```python
from build123d import *

# Parameters (mm, degrees)
BOSS_EXTRUDE1_DEPTH                                = 9.5
BOSS_EXTRUDE2_DEPTH                                = 2
BOSS_EXTRUDE4_DEPTH                                = 11.5
BOSS_EXTRUDE6_DEPTH                                = 7.5
CUT_EXTRUDE1_DEPTH                                 = 2
CUT_EXTRUDE2_REACH                                 = 85.313
SKETCH9_W                                          = 10
SKETCH9_H                                          = 3
CHAMFER1_SIZE                                      = 1
CHAMFER2_SIZE                                      = 1
CBORE_FOR_M2_5_PAN_HEAD_MACHINE_SCREW1_D           = 2.9
CBORE_FOR_M2_5_PAN_HEAD_MACHINE_SCREW1_CBORE_D     = 6
CBORE_FOR_M2_5_PAN_HEAD_MACHINE_SCREW1_CBORE_DEPTH = 2.1
CBORE_FOR_M2_5_PAN_HEAD_MACHINE_SCREW2_D           = 2.9
CBORE_FOR_M2_5_PAN_HEAD_MACHINE_SCREW2_CBORE_D     = 6
CBORE_FOR_M2_5_PAN_HEAD_MACHINE_SCREW2_CBORE_DEPTH = 2.1
CBORE_FOR_M2_5_PAN_HEAD_MACHINE_SCREW3_D           = 2.9
CBORE_FOR_M2_5_PAN_HEAD_MACHINE_SCREW3_CBORE_D     = 6
CBORE_FOR_M2_5_PAN_HEAD_MACHINE_SCREW3_CBORE_DEPTH = 2.1
CBORE_FOR_M2_5_PAN_HEAD_MACHINE_SCREW4_D           = 2.9
CBORE_FOR_M2_5_PAN_HEAD_MACHINE_SCREW4_CBORE_D     = 6
CBORE_FOR_M2_5_PAN_HEAD_MACHINE_SCREW4_CBORE_DEPTH = 2.1
SKETCH18_W                                         = 54.5
SKETCH18_H                                         = 7.531088913
CUT_EXTRUDE3_DEPTH                                 = 2


with BuildPart() as part:
    # Sketch2 → Boss-Extrude1 (new body)
    with BuildSketch(Plane(origin=(0, 0, 0), x_dir=(1, 0, 0), z_dir=(0, 1, 0))):
        with BuildLine():
            Line((-30.346153846, 41.446848386), (27.653846154, 41.446848386))
            ThreePointArc((27.653846154, 41.446848386), (32.250040232, 39.543042463), (34.153846154, 34.946848386))
            Line((34.153846154, 34.946848386), (34.153846154, -34.053151614))
            ThreePointArc((34.153846154, -34.053151614), (32.250040232, -38.649345692), (27.653846154, -40.553151614))
            Line((27.653846154, -40.553151614), (-30.346153846, -40.553151614))
            ThreePointArc((-30.346153846, -40.553151614), (-34.942347924, -38.649345692), (-36.846153846, -34.053151614))
            Line((-36.846153846, -34.053151614), (-36.846153846, 34.946848386))
            ThreePointArc((-36.846153846, 34.946848386), (-34.942347924, 39.543042463), (-30.346153846, 41.446848386))
        make_face()
        with BuildLine():
            Line((-30.346153846, 39.446848386), (27.653846154, 39.446848386))
            ThreePointArc((27.653846154, 39.446848386), (30.835826669, 38.128828901), (32.153846154, 34.946848386))
            Line((32.153846154, 34.946848386), (32.153846154, -34.053151614))
            ThreePointArc((32.153846154, -34.053151614), (30.835826669, -37.23513213), (27.653846154, -38.553151614))
            Line((27.653846154, -38.553151614), (-30.346153846, -38.553151614))
            ThreePointArc((-30.346153846, -38.553151614), (-33.528134361, -37.23513213), (-34.846153846, -34.053151614))
            Line((-34.846153846, -34.053151614), (-34.846153846, 34.946848386))
            ThreePointArc((-34.846153846, 34.946848386), (-33.528134361, 38.128828901), (-30.346153846, 39.446848386))
        make_face(mode=Mode.SUBTRACT)
    extrude(amount=BOSS_EXTRUDE1_DEPTH)

    # Sketch3 → Boss-Extrude2 (add)
    with BuildSketch(Plane(origin=(0, 0, 0), x_dir=(1, 0, 0), z_dir=(0, 1, 0))):
        with BuildLine():
            Line((-30.346153846, -38.553151614), (27.653846154, -38.553151614))
            ThreePointArc((27.653846154, -38.553151614), (30.835826669, -37.23513213), (32.153846154, -34.053151614))
            Line((32.153846154, -34.053151614), (32.153846154, 34.946848386))
            ThreePointArc((32.153846154, 34.946848386), (30.835826669, 38.128828901), (27.653846154, 39.446848386))
            Line((27.653846154, 39.446848386), (-30.346153846, 39.446848386))
            ThreePointArc((-30.346153846, 39.446848386), (-33.528134361, 38.128828901), (-34.846153846, 34.946848386))
            Line((-34.846153846, 34.946848386), (-34.846153846, -34.053151614))
            ThreePointArc((-34.846153846, -34.053151614), (-33.528134361, -37.23513213), (-30.346153846, -38.553151614))
        make_face()
    extrude(amount=BOSS_EXTRUDE2_DEPTH)

    # Sketch6 → Boss-Extrude4 (add)
    with BuildSketch(Plane(origin=(0, 2, 0), x_dir=(1, 0, 0), z_dir=(0, 1, 0))):
        with BuildLine():
            Line((-26.846153846, 34.946848386), (-26.846153846, 39.446848386))
            Line((-26.846153846, 39.446848386), (-30.346153846, 39.446848386))
            ThreePointArc((-30.346153846, 39.446848386), (-33.528134361, 38.128828901), (-34.846153846, 34.946848386))
            Line((-34.846153846, 34.946848386), (-34.846153846, 31.446848386))
            Line((-34.846153846, 31.446848386), (-30.346153846, 31.446848386))
            ThreePointArc((-30.346153846, 31.446848386), (-27.871280112, 32.471974652), (-26.846153846, 34.946848386))
        make_face()
        with BuildLine():
            Line((24.153846154, 34.946848386), (24.153846154, 39.446848386))
            Line((24.153846154, 39.446848386), (27.653846154, 39.446848386))
            ThreePointArc((27.653846154, 39.446848386), (30.835826669, 38.128828901), (32.153846154, 34.946848386))
            Line((32.153846154, 34.946848386), (32.153846154, 31.446848386))
            Line((32.153846154, 31.446848386), (27.653846154, 31.446848386))
            ThreePointArc((27.653846154, 31.446848386), (25.17897242, 32.471974652), (24.153846154, 34.946848386))
        make_face()
    extrude(amount=BOSS_EXTRUDE4_DEPTH)

    # Sketch8 → Boss-Extrude6 (add)
    with BuildSketch(Plane(origin=(0, 2, 0), x_dir=(1, 0, 0), z_dir=(0, 1, 0))):
        with BuildLine():
            Line((32.153846154, -30.553151614), (32.153846154, -34.053151614))
            ThreePointArc((32.153846154, -34.053151614), (30.835826669, -37.23513213), (27.653846154, -38.553151614))
            Line((27.653846154, -38.553151614), (24.153846154, -38.553151614))
            Line((24.153846154, -38.553151614), (24.153846154, -34.053151614))
            ThreePointArc((24.153846154, -34.053151614), (25.17897242, -31.57827788), (27.653846154, -30.553151614))
            Line((27.653846154, -30.553151614), (32.153846154, -30.553151614))
        make_face()
        with BuildLine():
            Line((-34.846153846, -30.553151614), (-34.846153846, -34.053151614))
            ThreePointArc((-34.846153846, -34.053151614), (-33.528134361, -37.23513213), (-30.346153846, -38.553151614))
            Line((-30.346153846, -38.553151614), (-26.846153846, -38.553151614))
            Line((-26.846153846, -38.553151614), (-26.846153846, -34.053151614))
            ThreePointArc((-26.846153846, -34.053151614), (-27.871280112, -31.57827788), (-30.346153846, -30.553151614))
            Line((-30.346153846, -30.553151614), (-34.846153846, -30.553151614))
        make_face()
    extrude(amount=BOSS_EXTRUDE6_DEPTH)

    # Sketch7 → Cut-Extrude1 (cut)
    with BuildSketch(Plane.XY.offset(40.553151614)):
        with BuildLine():
            Line((27.653846154, 9.5), (-30.346153846, 9.5))
            Line((-30.346153846, 9.5), (-26.595001855, 5.748848009))
            Line((-26.595001855, 5.748848009), (-22.39693017, 5.748848009))
            add(Edge.make_bspline(
                [(-22.39693017, 5.748848009), (-22.318478092, 3.867695791), (-21.39693017, 2.748848009)],
                knots=[0, 0, 0, 0.447396811, 0.447396811, 0.447396811], degree=2))
            Line((-21.39693017, 2.748848009), (-16.39693017, 2.748848009))
            add(Edge.make_bspline(
                [(-15.39693017, 5.748848009), (-15.475382247, 3.867695791), (-16.39693017, 2.748848009)],
                knots=[0, 0, 0, 0.447396811, 0.447396811, 0.447396811], degree=2))
            Line((-15.39693017, 5.748848009), (12.704622477, 5.748848009))
            add(Edge.make_bspline(
                [(12.704622477, 5.748848009), (12.783074555, 3.867695791), (13.704622477, 2.748848009)],
                knots=[0, 0, 0, 0.447396811, 0.447396811, 0.447396811], degree=2))
            Line((13.704622477, 2.748848009), (18.704622477, 2.748848009))
            add(Edge.make_bspline(
                [(19.704622477, 5.748848009), (19.6261704, 3.867695791), (18.704622477, 2.748848009)],
                knots=[0, 0, 0, 0.447396811, 0.447396811, 0.447396811], degree=2))
            Line((19.704622477, 5.748848009), (23.902694163, 5.748848009))
            Line((23.902694163, 5.748848009), (27.653846154, 9.5))
        make_face()
    extrude(amount=-CUT_EXTRUDE1_DEPTH, mode=Mode.SUBTRACT)

    # Sketch9 → Cut-Extrude2 (cut, up to next)
    with BuildSketch(Plane.ZY.offset(36.846153846), mode=Mode.PRIVATE) as cut_extrude2_sk1:
        with Locations((10.60615222, 8.033769059)):
            Rectangle(SKETCH9_W, SKETCH9_H)
    cut_extrude2_tool1 = extrude(cut_extrude2_sk1.sketch, amount=-CUT_EXTRUDE2_REACH, mode=Mode.PRIVATE) & part.part
    add(cut_extrude2_tool1.solids().sort_by_distance((-36.846154, 8.033769, 10.606152))[0], mode=Mode.SUBTRACT)

    # Chamfer1
    chamfer1_edges = [part.edges().sort_by_distance(p)[0] for p in [
        (-36.846153846, 8.01688453, 15.60615222),
        (-36.846153846, 8.01688453, 5.60615222),
        (-36.846153846, 6.533769059, 10.60615222),
    ]]
    chamfer(chamfer1_edges, length=CHAMFER1_SIZE)

    # Chamfer2
    chamfer2_edges = [part.edges().sort_by_distance(p)[0] for p in [
        (-36.846153846, 0, -0.446848386),
        (-34.942347924, 0, -39.543042463),
        (-1.346153846, 0, -41.446848386),
        (32.250040232, 0, -39.543042463),
        (34.153846154, 0, -0.446848386),
        (32.250040232, 0, 38.649345692),
        (-1.346153846, 0, 40.553151614),
        (-34.942347924, 0, 38.649345692),
    ]]
    chamfer(chamfer2_edges, length=CHAMFER2_SIZE)

    # CBORE for M2.5 Pan Head Machine Screw1 (through all)
    with Locations(Plane(origin=(0, 0, 0), x_dir=(-1, 0, 0), z_dir=(0, -1, 0))):
        with Locations((-27.653846154, 34.946848386)):
            CounterBoreHole(CBORE_FOR_M2_5_PAN_HEAD_MACHINE_SCREW1_D / 2, CBORE_FOR_M2_5_PAN_HEAD_MACHINE_SCREW1_CBORE_D / 2, CBORE_FOR_M2_5_PAN_HEAD_MACHINE_SCREW1_CBORE_DEPTH)

    # CBORE for M2.5 Pan Head Machine Screw2 (through all)
    with Locations(Plane(origin=(0, 0, 0), x_dir=(-1, 0, 0), z_dir=(0, -1, 0))):
        with Locations((30.346153846, 34.946848386)):
            CounterBoreHole(CBORE_FOR_M2_5_PAN_HEAD_MACHINE_SCREW2_D / 2, CBORE_FOR_M2_5_PAN_HEAD_MACHINE_SCREW2_CBORE_D / 2, CBORE_FOR_M2_5_PAN_HEAD_MACHINE_SCREW2_CBORE_DEPTH)

    # CBORE for M2.5 Pan Head Machine Screw3 (through all)
    with Locations(Plane(origin=(0, 0, 0), x_dir=(-1, 0, 0), z_dir=(0, -1, 0))):
        with Locations((-27.653846154, -34.053151614)):
            CounterBoreHole(CBORE_FOR_M2_5_PAN_HEAD_MACHINE_SCREW3_D / 2, CBORE_FOR_M2_5_PAN_HEAD_MACHINE_SCREW3_CBORE_D / 2, CBORE_FOR_M2_5_PAN_HEAD_MACHINE_SCREW3_CBORE_DEPTH)

    # CBORE for M2.5 Pan Head Machine Screw4 (through all)
    with Locations(Plane(origin=(0, 0, 0), x_dir=(-1, 0, 0), z_dir=(0, -1, 0))):
        with Locations((30.346153846, -34.053151614)):
            CounterBoreHole(CBORE_FOR_M2_5_PAN_HEAD_MACHINE_SCREW4_D / 2, CBORE_FOR_M2_5_PAN_HEAD_MACHINE_SCREW4_CBORE_D / 2, CBORE_FOR_M2_5_PAN_HEAD_MACHINE_SCREW4_CBORE_DEPTH)

    # Sketch18 → Cut-Extrude3 (cut)
    with BuildSketch(Plane(origin=(0, 9.5, 0), x_dir=(1, 0, 0), z_dir=(0, 1, 0))):
        with Locations((-1.346153846, -34.787607158)):
            Rectangle(SKETCH18_W, SKETCH18_H)
    extrude(amount=-CUT_EXTRUDE3_DEPTH, mode=Mode.SUBTRACT)


solid = part.part
```
Source: CAD feature listing. Evaluate the final solid. Frame: model axes, mm. A direction names the side the tool comes from. Give positions to 0.01 mm unless a question says otherwise; leave off trailing zeros. Loops run counter-clockwise (first coordinate to the right, second up) from the corner with the lowest first, then second, coordinate; pieces in that order, holes last. Notation, with made-up numbers: (88.25, 1.5) -> (117.25, 1.5) arc R13 ccw to (117.25, 24.5) -> close; hole circle Ø7 at (-4.5, 20.5). An arc over 180 degrees is marked (long way). Put each result on its own line as item: value. Start each with the question number.
1) Cut plane A-A (z = 2). Return loops of the section in (x, y), then the cut area to 3 significant figures.
2) Contact query for flat-ended pins moving along their axis: P1, Ø21.5, axis at x = 4, z = 12.5, coming from the +Y side; P2, Ø1.4, axis at x = 25, z = 36, coming from the +Y side; P3, Ø1, axis at x = 4.5, y = 6.5, coming from the +Z side. Output: stop coordinate, or through.
3) Material intervals for probe 1 along Z at (x, y) = (12, 4.5); probe 2 along X at (y, z) = (3.5, 11); probe 3 along Z at (x, y) = (28.5, 9), sorted ascending.
4) Reachability of faces 1 (the face through (-29, 11, -39.447)), 2 (the face through (-34.846, 11, -33)), 3 (the face through (24.154, 8, -37)) from +Z, -Z, +X, -X, +Y, -Y: full face, straight path, thin tool, end or side. Return the list, or none.
5) Cut plane B-B (x = 16.5). Return loops of the section in (y, z).
6) Cut plane C-C (y = 4). State how many separate pieces and enclosed holes the cut face has, then the cut area to 3 significant figures.
Results are:
1. outline: (-36.85, 1) -> (-35.85, 0) -> (33.15, 0) -> (34.15, 1) -> (34.15, 9.5) -> (32.15, 9.5) -> (32.15, 2) -> (-34.85, 2) -> (-34.85, 9.5) -> (-36.85, 9.5) -> close
1. area: 171 mm2
2. P1: stops at y = 2
2. P2: stops at y = 7.5
2. P3: stops at z = -39.45
3. probe 1: z = -41.45 to -39.45, 38.55 to 40.55
3. probe 2: x = -36.85 to -34.85, 32.15 to 34.15
3. probe 3: z = -41.39 to -36.12, -33.77 to -31.45, 30.55 to 32.88, 35.23 to 40.5
4. face 1: -Z, +X, -X, +Y
4. face 2: +Z, -Z, -X, +Y
4. face 3: +Y
5. outline: (0, -40.45) -> (1, -41.45) -> (9.5, -41.45) -> (9.5, -39.45) -> (2, -39.45) -> (2, 38.55) -> (2.75, 38.55) -> (2.75, 40.55) -> (1, 40.55) -> (0, 39.55) -> close
6. separate pieces: 2
6. enclosed holes: 4
6. area: 753 mm2
